```python
from build123d import *

# Parameters (mm, degrees)
SKETCH1_W           = 4.2
SKETCH1_H           = 8.6
SKETCH1_H_2         = 4.2
SKETCH1_R           = 1.25
BOSS_EXTRUDE1_DEPTH = 2.5


with BuildPart() as part:
    # Sketch1 → Boss-Extrude1 (new body)
    # profile 1 of 7: a face of its own
    with BuildSketch(Plane(origin=(0, 0, 0), x_dir=(1, 0, 0), z_dir=(0, 1, 0))):
        Polygon((-15.8, 8.5), (-15.8, 4.3), (-15.8, -4.3), (-15.8, -8.5), (15.8, -8.5), (15.8, -4.3), (15.8, 4.3), (15.8, 8.5), align=None)
    # profile 2 of 7: a face of its own
    with BuildSketch(Plane(origin=(0, 0, 0), x_dir=(1, 0, 0), z_dir=(0, 1, 0))):
        with Locations((-17.9, 0)):
            Rectangle(SKETCH1_W, SKETCH1_H)
    # profile 3 of 7: a face of its own
    with BuildSketch(Plane(origin=(0, 0, 0), x_dir=(1, 0, 0), z_dir=(0, 1, 0))):
        with Locations((-17.9, -6.4)):
            Rectangle(SKETCH1_W, SKETCH1_H_2)
        with Locations(Location((-17.9, -6.4, 0), (0, 0, 270))):
            Circle(SKETCH1_R, mode=Mode.SUBTRACT)
    # profile 4 of 7: a face of its own
    with BuildSketch(Plane(origin=(0, 0, 0), x_dir=(1, 0, 0), z_dir=(0, 1, 0))):
        with Locations((17.9, 6.4)):
            Rectangle(SKETCH1_W, SKETCH1_H_2)
        with Locations(Location((17.9, 6.4, 0), (0, 0, 270))):
            Circle(SKETCH1_R, mode=Mode.SUBTRACT)
    # profile 5 of 7: a face of its own
    with BuildSketch(Plane(origin=(0, 0, 0), x_dir=(1, 0, 0), z_dir=(0, 1, 0))):
        with Locations((17.9, 0)):
            Rectangle(SKETCH1_W, SKETCH1_H)
    # profile 6 of 7: a face of its own
    with BuildSketch(Plane(origin=(0, 0, 0), x_dir=(1, 0, 0), z_dir=(0, 1, 0))):
        with Locations((17.9, -6.4)):
            Rectangle(SKETCH1_W, SKETCH1_H_2)
        with Locations(Location((17.9, -6.4, 0), (0, 0, 270))):
            Circle(SKETCH1_R, mode=Mode.SUBTRACT)
    # profile 7 of 7: a face of its own
    with BuildSketch(Plane(origin=(0, 0, 0), x_dir=(1, 0, 0), z_dir=(0, 1, 0))):
        with Locations((-17.9, 6.4)):
            Rectangle(SKETCH1_W, SKETCH1_H_2)
        with Locations(Location((-17.9, 6.4, 0), (0, 0, 270))):
            Circle(SKETCH1_R, mode=Mode.SUBTRACT)
    extrude(amount=BOSS_EXTRUDE1_DEPTH)


solid = part.part
```
Can you work these out from the model? Positions are in its coordinate system, mm. Round coordinates to 2 decimals unless told otherwise and drop trailing zeros. Loops run counter-clockwise (first coordinate to the right, second up) from the corner with the lowest first, then second, coordinate; pieces in that order, holes last. Notation, with made-up numbers: (-36, 6) -> (16, 6) arc R22 ccw to (16, 41) -> close; hole circle Ø2 at (40, 21.5). An arc over 180 degrees is marked (long way). Answer in a Markdown table with one row per item.
Item 1: Suppose I cut it at B-B, the plane x = 17.9. List the corners of the cut face in (y, z) for me.
Answer block:
| item | result |
|---|---|
| outline | (0, -8.5) -> (2.5, -8.5) -> (2.5, -7.65) -> (0, -7.65) -> close; (0, -5.15) -> (2.5, -5.15) -> (2.5, 5.15) -> (0, 5.15) -> close; (0, 7.65) -> (2.5, 7.65) -> (2.5, 8.5) -> (0, 8.5) -> close |
Item 2: We'd pull the mould along X, two halves only. Please class faces 1 (the flat face through (0, 1, -8.5)), 2 (the flat face through (20, 1, 0)), 3 (the cylindrical face through (-16.846, 1.232, 7.072)), 4 (the cylindrical face through (-16.846, 1.232, -5.728)): released by +X, released by -X, zero draft, split by the parting line, or undercut.
Answer block:
| item | result |
|---|---|
| face 1 | zero draft |
| face 2 | released by +X |
| face 3 | undercut |
| face 4 | undercut |
Item 3: If I drill on probe 1 along X at (y, z) = (1.9, 6.4); probe 2 along Z at (x, y) = (18.5, 0.25); probe 3 along X at (y, z) = (0.5, 7), over which ranges is the centre line in solid material (lowest first)?
Answer block:
| item | result |
|---|---|
| probe 1 | -20 to -19.15, -16.65 to 16.65, 19.15 to 20 |
| probe 2 | -8.5 to -7.5, -5.3 to 5.3, 7.5 to 8.5 |
| probe 3 | -20 to -19, -16.8 to 16.8, 19 to 20 |
Item 4: Suppose I cut it at A-A, the plane z = 6.4. List the corners of the cut face in (x, y) for me, plus the area to 3 significant figures.
Answer block:
| item | result |
|---|---|
| outline | (-20, 0) -> (-19.15, 0) -> (-19.15, 2.5) -> (-20, 2.5) -> close; (-16.65, 0) -> (16.65, 0) -> (16.65, 2.5) -> (-16.65, 2.5) -> close; (19.15, 0) -> (20, 0) -> (20, 2.5) -> (19.15, 2.5) -> close |
| area | 87.5 mm² |
Item 5: Will this pin go through, and if not, where does the flat tip stop? P1, Ø3, axis at x = 17.9, z = -6.4, coming from the -Y side.
Answer block:
| item | result |
|---|---|
| P1 | y = 0 |
Item 6: Suppose I cut it at C-C, the plane y = 1.4. List the corners of the cut face in (x, z) for me, plus the area to 3 significant figures.
Answer block:
| item | result |
|---|---|
| outline | (-20, -8.5) -> (20, -8.5) -> (20, 8.5) -> (-20, 8.5) -> close; hole circle Ø2.5 at (-17.9, -6.4); hole circle Ø2.5 at (-17.9, 6.4); hole circle Ø2.5 at (17.9, -6.4); hole circle Ø2.5 at (17.9, 6.4) |
| area | 660 mm² |
